Source: CAD feature listing. Evaluate the final solid. Frame: model axes, mm. Face numbers are marked on the shaded views. A direction names the side the tool comes from. Round coordinates to 2 decimals unless told otherwise and drop trailing zeros. Loops run counter-clockwise (first coordinate to the right, second up) from the corner with the lowest first, then second, coordinate; pieces in that order, holes last. Notation, with made-up numbers: M 10,-27 L 17,-27 A15 cw 17,-18 Z; hole C -18,4 d5. An arc over 180 degrees is marked long. Answer as a JSON object with one key per item and string values.
from build123d import *

# Parameters (mm, degrees)
BOSS_EXTRUDE1_DEPTH = 52
BOSS_EXTRUDE2_DEPTH = 4.5
CUT_EXTRUDE1_REACH  = 84.366
SKETCH3_W           = 60
SKETCH3_H           = 39.2
CUT_EXTRUDE2_REACH  = 84.366
SKETCH4_W           = 49
SKETCH4_H           = 12


with BuildPart() as part:
    # Sketch1 → Boss-Extrude1 (new body)
    with BuildSketch(Plane(origin=(0, 0, 0), x_dir=(1, 0, 0), z_dir=(0, 1, 0))):
        with BuildLine():
            Line((-42.95, -9.9), (-42.95, 14.309085823))
            Line((-42.95, 14.309085823), (-31.436935022, 20.9))
            Line((-31.436935022, 20.9), (31.436935022, 20.9))
            Line((31.436935022, 20.9), (42.95, 14.309085823))
            Line((42.95, 14.309085823), (42.95, -9.9))
            ThreePointArc((42.95, -9.9), (39.728174593, -17.678174593), (31.95, -20.9))
            Line((31.95, -20.9), (-31.95, -20.9))
            ThreePointArc((-31.95, -20.9), (-39.728174593, -17.678174593), (-42.95, -9.9))
        make_face()
        with BuildLine():
            Line((-38.45, 11.7), (-30.24, 16.4))
            Line((-30.24, 16.4), (30.24, 16.4))
            Line((30.24, 16.4), (38.45, 11.7))
            Line((38.45, 11.7), (38.45, -9.9))
            ThreePointArc((38.45, -9.9), (36.546194078, -14.496194078), (31.95, -16.4))
            Line((31.95, -16.4), (-31.95, -16.4))
            ThreePointArc((-31.95, -16.4), (-36.546194078, -14.496194078), (-38.45, -9.9))
            Line((-38.45, -9.9), (-38.45, 11.7))
        make_face(mode=Mode.SUBTRACT)
    extrude(amount=BOSS_EXTRUDE1_DEPTH)

    # Sketch2 → Boss-Extrude2 (add)
    with BuildSketch(Plane(origin=(0, 52, 0), x_dir=(1, 0, 0), z_dir=(0, 1, 0))):
        with BuildLine():
            Line((-31.95, -20.9), (31.95, -20.9))
            ThreePointArc((31.95, -20.9), (39.728174593, -17.678174593), (42.95, -9.9))
            Line((42.95, -9.9), (42.95, 14.309085823))
            Line((42.95, 14.309085823), (31.436935022, 20.9))
            Line((31.436935022, 20.9), (-31.436935022, 20.9))
            Line((-31.436935022, 20.9), (-42.95, 14.309085823))
            Line((-42.95, 14.309085823), (-42.95, -9.9))
            ThreePointArc((-42.95, -9.9), (-39.728174593, -17.678174593), (-31.95, -20.9))
        make_face()
    extrude(amount=BOSS_EXTRUDE2_DEPTH)

    # Sketch3 → Cut-Extrude1 (cut, up to next)
    with BuildSketch(Plane.XY.offset(20.9), mode=Mode.PRIVATE) as cut_extrude1_sk1:
        with Locations((0, 19.6)):
            Rectangle(SKETCH3_W, SKETCH3_H)
    cut_extrude1_tool1 = extrude(cut_extrude1_sk1.sketch, amount=-CUT_EXTRUDE1_REACH, mode=Mode.PRIVATE) & part.part
    add(cut_extrude1_tool1.solids().sort_by_distance((0, 19.6, 20.9))[0], mode=Mode.SUBTRACT)

    # Sketch4 → Cut-Extrude2 (cut, up to next)
    with BuildSketch(Plane(origin=(0, 0, -20.9), x_dir=(-1, 0, 0), z_dir=(0, 0, -1)), mode=Mode.PRIVATE) as cut_extrude2_sk1:
        with Locations((0, 6)):
            Rectangle(SKETCH4_W, SKETCH4_H)
    cut_extrude2_tool1 = extrude(cut_extrude2_sk1.sketch, amount=-CUT_EXTRUDE2_REACH, mode=Mode.PRIVATE) & part.part
    add(cut_extrude2_tool1.solids().sort_by_distance((0, 6, -20.9))[0], mode=Mode.SUBTRACT)


solid = part.part
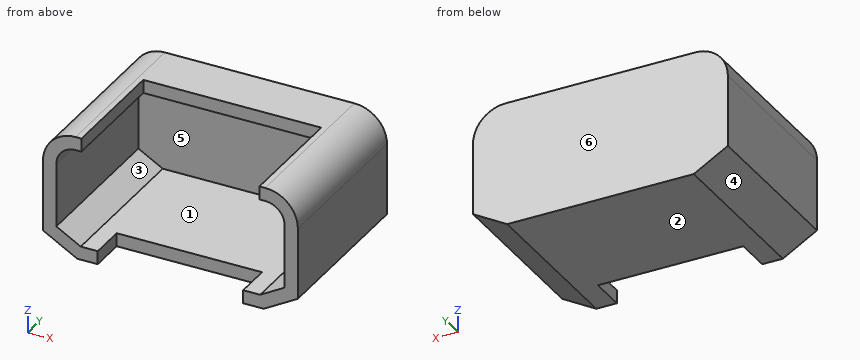
Item 1: Access query for the marked faces 1 and 2. Directions: +Z, -Z, +X, -X, +Y, -Y. A direction counts if a zero-diameter tool reaches every point of the face in a straight line with its end or side. Return the directions, or none.
Answer sheet:
{"face 1": "-Y", "face 2": "-Z, +X, -X, +Y, -Y"}
Item 2: Section A-A on x = -29. Return the cut outline in (y, z), then the cut area to 3 significant figures.
Answer sheet:
{"outline": "M 0,-20.9 L 56.5,-20.9 L 56.5,20.9 L 39.2,20.9 L 39.2,16.4 L 52,16.4 L 52,-16.4 L 0,-16.4 Z", "area": "480 mm²"}
Item 3: Contact query for flat-ended pins moving along their axis: pin 1 Ø5 at (y, z) = (13.5, 19) entering from +X; pin 2 Ø15.5 at (x, y) = (-7, 24) entering from +Z; pin 3 Ø3.5 at (x, z) = (7, 19.5) entering from -Y. Output: stop coordinate, or through.
Answer sheet:
{"pin 1": "stops at x = 40.75", "pin 2": "stops at z = -16.4", "pin 3": "stops at y = 39.2"}
Item 4: Line query: probe 1 along X at (y, z) = (13.5, 9); probe 2 along Z at (x, y) = (18.5, 35.5); probe 3 along Z at (x, y) = (-25, 50). Output: solid intervals per line, ascending. Write a range as from..to.
Answer sheet:
{"probe 1": "x = -42.95..-38.45, 38.45..42.95", "probe 2": "z = -20.9..-16.4", "probe 3": "z = -20.9..-16.4, 16.4..20.9"}
Item 5: Section C-C on y = 18. Return the cut outline in (x, z), then the cut area to 3 significant figures.
Answer sheet:
{"outline": "M -42.95,-14.31 L -31.44,-20.9 L 31.44,-20.9 L 42.95,-14.31 L 42.95,9.9 A11 ccw 31.95,20.9 L 30,20.9 L 30,16.4 L 31.95,16.4 A6.5 cw 38.45,9.9 L 38.45,-11.7 L 30.24,-16.4 L -30.24,-16.4 L -38.45,-11.7 L -38.45,9.9 A6.5 cw -31.95,16.4 L -30,16.4 L -30,20.9 L -31.95,20.9 A11 ccw -42.95,9.9 Z", "area": "727 mm²"}
Item 6: Section B-B on y = 48.5. Return the cut outline in (x, z).
Answer sheet:
{"outline": "M -42.95,-14.31 L -31.44,-20.9 L 31.44,-20.9 L 42.95,-14.31 L 42.95,9.9 A11 ccw 31.95,20.9 L -31.95,20.9 A11 ccw -42.95,9.9 Z; hole M -38.45,-11.7 L -30.24,-16.4 L 30.24,-16.4 L 38.45,-11.7 L 38.45,9.9 A6.5 ccw 31.95,16.4 L -31.95,16.4 A6.5 ccw -38.45,9.9 Z"}
Item 7: Section D-D on z = 1. Return the cut outline in (x, y).
Answer sheet:
{"outline": "M -42.95,0 L -38.45,0 L -38.45,52 L 38.45,52 L 38.45,0 L 42.95,0 L 42.95,56.5 L -42.95,56.5 Z"}
Item 8: Pull-direction query (Z, two-part tool) for the marked faces 3, 4, 5 and 6; classes: pulls with the +Z half, pulls with the -Z half, needs draft (parallel to the pull), parting line crosses it, or undercut.
Answer sheet:
{"face 3": "undercut", "face 4": "pulls with the -Z half", "face 5": "undercut", "face 6": "needs draft"}
